Design review of the part shown in the three views and the two pictorial views. Dimensions are in mm from the part's minimum x, y and z. Coordinates: 2 decimals unless noted, no trailing zeros. Write each loop counter-clockwise with the first axis right and the second up, starting at its lowest first coordinate (ties: lowest second). Pieces come first, ordered by that corner, then holes.
Q1. For L1, parallel to Y at x = 196.2, z = 13.35; L2, parallel to X at y = 16, z = 5.5; L3, parallel to X at y = 36, z = 13.5, list the stretches that pass through material, from the lowest coordinate up.
Q2. Take a section at A-A, the plane y = 17. Write out the cut boundary in (x, z).
Q3. For pin 1 Ø5 at (y, z) = (30, 7) entering from +X; pin 2 Ø5 at (y, z) = (4.5, 2.5) entering from -X; pin 3 Ø6 at (x, y) = (5, 12) entering from -Z, all flat-tipped, find the tip position at first contact; note any pin that passes through.
Q4. The part is to be moulded in two halves that separate along X. For the marked faces 1 and 2, say which applies: released by +X, released by -X, zero draft, split by the parting line, or undercut.
Q5. Take a section at B-B, the plane x = 125.5. Write out the cut boundary in (y, z).
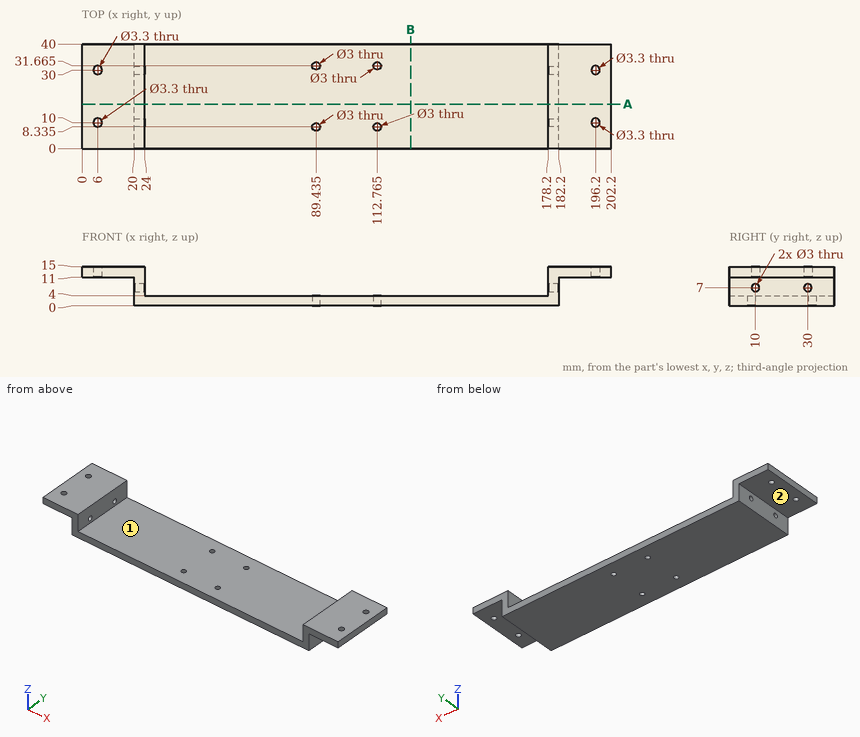
Responses:
1. L1: y = 0 to 8.35, 11.65 to 28.35, 31.65 to 40
1. L2: x = 20 to 24, 178.2 to 182.2
1. L3: x = 0 to 24, 178.2 to 202.2
2. outline: (0, 11) - (20, 11) - (20, 0) - (182.2, 0) - (182.2, 11) - (202.2, 11) - (202.2, 15) - (178.2, 15) - (178.2, 4) - (24, 4) - (24, 15) - (0, 15) - close
3. pin 1: stops at x = 182.2
3. pin 2: stops at x = 20
3. pin 3: stops at z = 11
4. face 1: undercut
4. face 2: zero draft
5. outline: (0, 0) - (40, 0) - (40, 4) - (0, 4) - close
